from build123d import *

# Parameters (mm, degrees)
F0_W     = 19.05
F0_H     = 57.15
F1_DEPTH = 457.2
F2_W     = 19.05
F2_H     = 28.575
F3_DEPTH = 19.05
F4_R     = 50.8


with BuildPart() as f1:
    # F0 (on Front) → F1 (new body)
    with BuildSketch(Plane.XZ):
        with Locations((9.525, 28.575)):
            Rectangle(F0_W, F0_H)
    extrude(amount=F1_DEPTH)

    # F2 (on face) → F3 (cut, through all)
    with BuildSketch(Plane.YZ.offset(19.05)):
        with Locations((-228.6, 42.8625)):
            Rectangle(F2_W, F2_H)
    extrude(amount=-F3_DEPTH, mode=Mode.SUBTRACT)

    # F4
    f4_edges = [f1.edges().sort_by_distance(p)[0] for p in [
        (9.525, 0, 57.15),
        (9.525, -457.2, 57.15),
    ]]
    fillet(f4_edges, radius=F4_R)


solid = f1.part
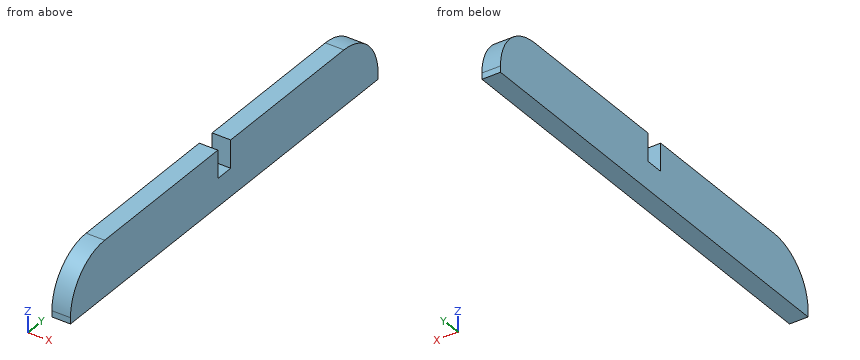
Input: part model. Units: mm. Frame: model coordinates. Round coordinates to 2 decimals unless told otherwise and drop trailing zeros. Order: outer loops, then holes, each group sorted by start corner. A loop starts at its lowest first (then second) coordinate and runs counter-clockwise, first axis right, second up. Notation, with made-up numbers: (79, 61.25) - (127, 61.25) arc R20 cw to (127, 97.25) - close; hole circle Ø6 at (2.25, 59.5). An arc over 180 degrees is marked (long way). Answer as a JSON object with one key per item and string values. Group by question number.
(1) Cut plane B-B (x = 13.25). Return loops of the section in (y, z) (3 decimals).
(2) Pin query (flat end, axial travel): P1, Ø9.5, axis at x = 11, z = 42.5, coming from the -Y side; P2, Ø8, axis at x = 9, z = 26, coming from the -Y side; P3, Ø3, axis at x = 8.5, z = 19.5, coming from the +Y side. Return the tip coordinate at first contact, or that it passes through.
(3) Cut plane A-A (z = 41.5). Return loops of the section in (x, y) (3 decimals), then the cut area to 3 significant figures.
(4) Material intervals for probe 1 along Y at (x, z) = (18.25, 35.5) (3 decimals); probe 2 along Y at (x, z) = (10.25, 52) (3 decimals); probe 3 along Y at (x, z) = (10, 9), sorted ascending. Write a range as from..to.
Here are the results:
{
 "1": {"outline": "(-457.2, 0) - (0, 0) - (0, 6.35) arc R50.8 ccw to (-50.8, 57.15) - (-219.075, 57.15) - (-219.075, 28.575) - (-238.125, 28.575) - (-238.125, 57.15) - (-406.4, 57.15) arc R50.8 ccw to (-457.2, 6.35) - close"},
 "2": {"P1": "stops at y = -446.33", "P2": "stops at y = -454.73", "P3": "stops at y = -1.35"},
 "3": {"outline": "(0, -443.076) - (19.05, -443.076) - (19.05, -238.125) - (0, -238.125) - close; (0, -219.075) - (19.05, -219.075) - (19.05, -14.124) - (0, -14.124) - close", "area": "7,810 mm^2"},
 "4": {"probe 1": "y = -448.004..-238.125, -219.075..-9.196", "probe 2": "y = -428.687..-238.125, -219.075..-28.513", "probe 3": "y = -457.13..-0.07"}
}
